Geometry check sheet. Reference: the model listing, model coordinates, mm. A direction names the side the tool comes from. Round coordinates to 2 decimals unless told otherwise and drop trailing zeros.
```python
from build123d import *

# Parameters (mm, degrees)
SKETCH2_R   = 4.7625
SKETCH2_R_2 = 3.175


with BuildPart() as part:
    # Sweep1: sweep along a path in Sketch1
    with BuildLine(Plane.XY) as sweep1_path:
        Line((0, 0), (0, 254))
        ThreePointArc((0, 254), (0.198630909, 260.362390256), (0.79375, 266.7))
        ThreePointArc((0.79375, 266.7), (1.388869091, 273.037609744), (1.5875, 279.4))
        Line((1.5875, 279.4), (1.5875, 527.05))
        ThreePointArc((1.5875, 527.05), (3.663854401, 537.377471366), (9.570241337, 546.1))
        ThreePointArc((9.570241337, 546.1), (15.476628273, 554.822528634), (17.552982674, 565.15))
        Line((17.552982674, 565.15), (17.552982674, 590.55))
    # Sketch2 → Sweep1 (sweep)
    with BuildSketch(Plane(origin=(0, 0, 0), x_dir=(1, 0, 0), z_dir=(0, 1, 0))):
        Circle(SKETCH2_R)
        Circle(SKETCH2_R_2, mode=Mode.SUBTRACT)
    sweep(path=sweep1_path.line)


solid = part.part
```
(1) Draft check along X on faces 3 (the flat face through (14, 590.55, 1)), 4 (the cylindrical face through (-3.78, 128.78, 2.9)). Enter one of: released by +X, released by -X, zero draft, split by the parting line, or undercut.
Returned:
face 3: zero draft
face 4: split by the parting line
(2) Set-up check for faces 1 (the cylindrical face through (21.952, 578.028, 1.824)), 2 (the cylindrical face through (-2.19, 404.96, 2.9)): record each of +Z, -Z, +X, -X, +Y, -Y from which the full face is reachable in a straight line by a thin tool's end or side.
Returned:
face 1: +Y
face 2: none
(3) Material ranges on line 1 (X direction, y = 582.5, z = 0); line 2 (Z direction, x = 2, y = 497); line 3 (Z direction, x = 0, y = 103.5) (1 decimal), recorded low to high.
Returned:
line 1: x = 12.79 to 14.38, 20.73 to 22.32
line 2: z = -4.74 to -3.15, 3.15 to 4.74
line 3: z = -4.8 to -3.2, 3.2 to 4.8
(4) Depth check by flat-ended pin: P1, Ø4, axis at y = 331, z = 0, coming from the -X side (3 decimals); P2, Ø5, axis at x = 18.5, z = -0.5, coming from the -Y side; P3, Ø1, axis at x = 15, z = 1, coming from the +Y side; P4, Ø10, axis at x = 13.5, y = 176.5, coming from the -Z side. Enter the tip coordinate at first touch or a pass-through.
Returned:
P1: stops at x = -3.175
P2: stops at y = 546.26
P3: stops at y = 590.55
P4: passes through
